Work out the finished part from the listing and answer in its coordinate system (mm). A direction names the side the tool comes from. Round coordinates to 2 decimals unless told otherwise and drop trailing zeros. Order: outer loops, then holes, each group sorted by start corner. A loop starts at its lowest first (then second) coordinate and runs counter-clockwise, first axis right, second up. Notation, with made-up numbers: (78, 67) - (102, 67) arc R14 ccw to (102, 94) - close; hole circle Ø7 at (-24, -40). An arc over 180 degrees is marked (long way). Put each result on its own line as item: value.
```python
from build123d import *

# Parameters (mm, degrees)
CROQUIS2_R            = 1.5
CORTAR_EXTRUIR1_DEPTH = 2


with BuildPart() as part:
    # Croquis1 → Revolución3 (revolve)
    with BuildSketch(Plane.XY):
        Polygon((0, 5), (0, -5), (7, -5), (4.172417728, -1.5), (4.172417728, 1.5), (7, 5), align=None)
    revolve(axis=Axis((0, 14.056584816, 0), (0, -1, 0)))

    # Croquis2 → Cortar-Extruir1 (cut)
    with BuildSketch(Plane(origin=(0, -5, 0), x_dir=(-1, 0, 0), z_dir=(0, -1, 0))):
        Circle(CROQUIS2_R)
    extrude(amount=-CORTAR_EXTRUIR1_DEPTH, mode=Mode.SUBTRACT)


solid = part.part
```
1) A cutting plane is placed at C-C on y = 1. Write down the section's boundary in (x, z).
Findings below:
outline: circle Ø8.34 at (0, 0)
2) Given pin 1 Ø3 at (x, y) = (-1.5, 1) entering from -Z; pin 2 Ø3 at (y, z) = (2, -3) entering from -X; pin 3 Ø1 at (y, z) = (1, 0.5) entering from +X, each flat-ended and moving along its own axis, determine where each tip first touches the part or whether it passes through.
Findings below:
pin 1: stops at z = -4.81
pin 2: stops at x = -5.16
pin 3: stops at x = 4.17
3) A cutting plane is placed at D-D on y = 4.25. Write down the section's boundary in (x, z), then the cut area to 3 significant figures.
Findings below:
outline: circle Ø12.79 at (0, 0)
area: 128 mm2
4) Straight lines are drawn through the part: L1, parallel to X at y = -4.15, z = 0; L2, parallel to X at y = -3.55, z = 0; L3, parallel to Z at x = 0, y = -4.4. For each, find the intervals that lie inside material, in ascending order. Write a range as from..to.
Findings below:
L1: x = -6.31..-1.5, 1.5..6.31
L2: x = -5.83..-1.5, 1.5..5.83
L3: z = -6.52..-1.5, 1.5..6.52
5) For faces 4 (the cylindrical face through (1.5, -4.01, -0.07)), 5 (the conical face through (4.15, 1.72, 1.31)), 6 (the flat face through (0, 5, 0)), determine the directions among +Z, -Z, +X, -X, +Y, -Y from which every point of the face is accessible in a straight line to the end or side of a thin tool.
Findings below:
face 4: -Y
face 5: none
face 6: +Z, -Z, +X, -X, +Y
6) A cutting plane is placed at B-B on x = 0. Write down the section's boundary in (y, z).
Findings below:
outline: (-5, -7) - (-1.5, -4.17) - (1.5, -4.17) - (5, -7) - (5, 7) - (1.5, 4.17) - (-1.5, 4.17) - (-5, 7) - (-5, 1.5) - (-3, 1.5) - (-3, -1.5) - (-5, -1.5) - close
7) For a pull along Z with two mould halves and no side action, classify faces 1 (the flat face through (0, -3, 0)), 2 (the flat face through (0, -5, 2)), 3 (the conical face through (4.11, -1.67, 1.29)) as pulls with the +Z half, pulls with the -Z half, needs draft (parallel to the pull), parting line crosses it, or undercut.
Findings below:
face 1: undercut
face 2: needs draft
face 3: parting line crosses it
8) A cutting plane is placed at A-A on z = 0. Write down the section's boundary in (x, y), then the cut area to 3 significant figures.
Findings below:
outline: (-7, -5) - (-1.5, -5) - (-1.5, -3) - (1.5, -3) - (1.5, -5) - (7, -5) - (4.17, -1.5) - (4.17, 1.5) - (7, 5) - (-7, 5) - (-4.17, 1.5) - (-4.17, -1.5) - close
area: 97.2 mm2
